Drawing for the job (mm, zero at the part's lowest x, y, z). A direction names the side the tool comes from. Coordinates: 2 decimals unless noted, no trailing zeros. Loops run counter-clockwise (first coordinate to the right, second up) from the corner with the lowest first, then second, coordinate; pieces in that order, holes last. Notation, with made-up numbers: (-11, -30.5) - (47, -30.5) arc R12 cw to (47, -17.5) - close; hole circle Ø8 at (36, 12). An arc over 180 degrees is marked (long way). Put each result on its own line as item: value.
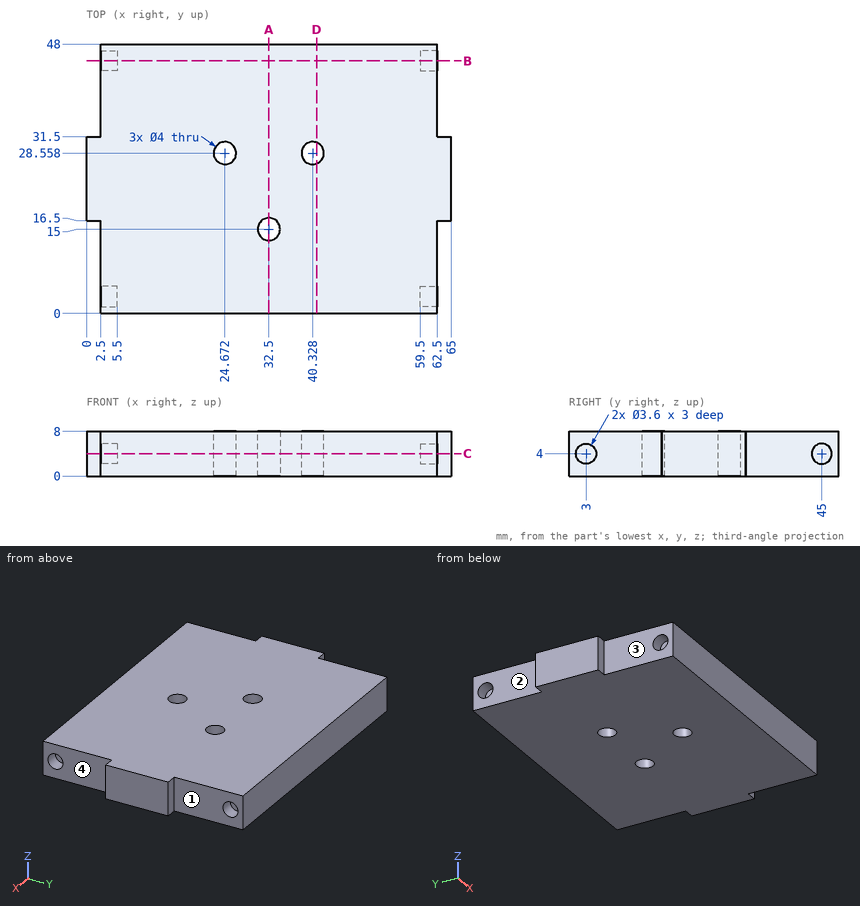
Q1. Wall check: L1, parallel to Z at x = 61, y = 3; L2, parallel to X at y = 10, z = 7; L3, parallel to X at y = 4, z = 5.25. Give the ranges that are in metal, low to high. Write a range as from..to.
Determined:
L1: 0..2.2, 5.8..8
L2: 2.5..62.5
L3: 5.5..59.5
Q2. Slice it at B-B, the plane y = 45. Give the cut face in (x, z).
Determined:
outline: (2.5, 0) - (62.5, 0) - (62.5, 2.2) - (59.5, 2.2) - (59.5, 5.8) - (62.5, 5.8) - (62.5, 8) - (2.5, 8) - (2.5, 5.8) - (5.5, 5.8) - (5.5, 2.2) - (2.5, 2.2) - close
Q3. Slice it at D-D, the plane x = 41. Give the cut face in (y, z) (1 decimal).
Determined:
outline: (0, 0) - (26.7, 0) - (26.7, 8) - (0, 8) - close; (30.4, 0) - (48, 0) - (48, 8) - (30.4, 8) - close
Q4. Pin check, flat tips, straight feed: pin 1 Ø4.5 at (y, z) = (45, 4) entering from -X; pin 2 Ø3 at (y, z) = (45, 4) entering from +X; pin 3 Ø4 at (y, z) = (45, 3.5) entering from +X. Stop position of each tip, or through.
Determined:
pin 1: x = 2.5
pin 2: x = 59.5
pin 3: x = 62.5
Q5. Slice it at A-A, the plane x = 32.5. Give the cut face in (y, z).
Determined:
outline: (0, 0) - (13, 0) - (13, 8) - (0, 8) - close; (17, 0) - (48, 0) - (48, 8) - (17, 8) - close
Q6. Tool access for the marked faces 1, 2, 3 and 4: list every direction of +Z, -Z, +X, -X, +Y, -Y with a clear straight run to the whole face (end or side of a thin tool).
Determined:
face 1: +Z, -Z, +X, +Y
face 2: +Z, -Z, -X, +Y
face 3: +Z, -Z, -X, -Y
face 4: +Z, -Z, +X, -Y
Q7. Slice it at C-C, the plane z = 4. State how many separate pieces and enclosed holes the cut face has, then the cut area to 3 significant figures.
Determined:
separate pieces: 1
enclosed holes: 3
area: 2,870 mm2
